from build123d import *

# Parameters (mm, degrees)
SALIENTE_EXTRUIR1_DEPTH  = 67.25
CROQUIS7_R               = 4
SALIENTE_EXTRUIR2_DEPTH  = 15
SALIENTE_EXTRUIR9_DEPTH  = 7.5
CROQUIS15_R              = 4
SALIENTE_EXTRUIR15_DEPTH = 9
CROQUIS17_W              = 25
CROQUIS17_H              = 5
SALIENTE_EXTRUIR16_DEPTH = 17.5
CROQUIS18_R              = 1.75
CORTAR_EXTRUIR3_DEPTH    = 7.5


with BuildPart() as part:
    # Croquis2 → Saliente-Extruir1 (new body)
    with BuildSketch(Plane(origin=(0, 0, 0), x_dir=(1, 0, 0), z_dir=(0, 1, 0))):
        Polygon((-17.5, -27.121137051), (17.5, -27.121137051), (17.5, -17.121137051), (9.5, -17.121137051), (9.5, -14.121137051), (17.5, -14.121137051), (7.5, -4.121137051), (-7.5, -4.121137051), (-17.5, -14.121137051), (-9.5, -14.121137051), (-9.5, -17.121137051), (-17.5, -17.121137051), align=None)
    extrude(amount=SALIENTE_EXTRUIR1_DEPTH)

    # Croquis7 → Saliente-Extruir2 (add)
    with BuildSketch(Plane.XY.offset(27.121137051)):
        with Locations(Location((0, 54.15, 0), (0, 0, 180))):
            Circle(CROQUIS7_R)
    extrude(amount=SALIENTE_EXTRUIR2_DEPTH)



with BuildPart() as body_2:
    # Croquis8 → Saliente-Extruir9 (new, symmetric)
    with BuildSketch(Plane(origin=(0, 0, 0), x_dir=(0, 0, -1), z_dir=(1, 0, 0))):
        Polygon((-36.121137051, 47.65), (-30.523413607, 47.65), (-27.121137051, 47.65), (-27.121137051, 37.610022974), align=None)
    extrude(amount=SALIENTE_EXTRUIR9_DEPTH, both=True)


with BuildPart() as part_1:
    add(part.part)

    add(body_2.part)  # Saliente-Extruir15 merges body 2
    # Croquis15 → Saliente-Extruir15 (add)
    with BuildSketch(Plane.XY.offset(27.121137051)):
        with BuildLine():
            Line((-7.5, 47.65), (7.5, 47.65))
            Line((7.5, 47.65), (7.5, 57.15))
            ThreePointArc((7.5, 57.15), (6.474873734, 59.624873734), (4, 60.65))
            Line((4, 60.65), (-4, 60.65))
            ThreePointArc((-4, 60.65), (-6.474873734, 59.624873734), (-7.5, 57.15))
            Line((-7.5, 57.15), (-7.5, 47.65))
        make_face()
        with Locations(Location((0, 54.15, 0), (0, 0, 180))):
            Circle(CROQUIS15_R, mode=Mode.SUBTRACT)
    extrude(amount=SALIENTE_EXTRUIR15_DEPTH)

    # Croquis17 → Saliente-Extruir16 (add, symmetric)
    with BuildSketch(Plane(origin=(0, 0, 0), x_dir=(0, 0, -1), z_dir=(1, 0, 0))):
        with Locations((-39.621137051, 5.5)):
            Rectangle(CROQUIS17_W, CROQUIS17_H)
    extrude(amount=SALIENTE_EXTRUIR16_DEPTH, both=True)

    # Croquis18 → Cortar-Extruir3 (cut, symmetric)
    with BuildSketch(Plane(origin=(0, 8, 0), x_dir=(1, 0, 0), z_dir=(0, 1, 0))):
        with Locations(Location((0, -47.121137051, 0), (0, 0, 270))):
            Circle(CROQUIS18_R)
    extrude(amount=CORTAR_EXTRUIR3_DEPTH, both=True, mode=Mode.SUBTRACT)


solid = part_1.part
Model file for the job. Use its own axes, mm. A direction names the side the tool comes from. Give positions to 0.01 mm unless a question says otherwise; leave off trailing zeros. Loops run counter-clockwise (first coordinate to the right, second up) from the corner with the lowest first, then second, coordinate; pieces in that order, holes last. Notation, with made-up numbers: (67.25, -21) -> (123.25, -21) arc R20 ccw to (123.25, -1) -> close; hole circle Ø6 at (-6, 86.25). An arc over 180 degrees is marked (long way). Use a Markdown table: item, result. Add a question column.
(1) Slice it at D-D on z = 44. List the corners of the cut face in (x, y).
(2) Tool access for faces 5 (the flat face through (0, 54, 42.121)), 6 (the flat face through (9.5, 33, 16)), 7 (the cylindrical face through (-6.4, 59.7, 31.6)): list every direction of +Z, -Z, +X, -X, +Y, -Y with a clear straight run to the whole face (end or side of a thin tool).
(3) Slice it at B-B on y = 54.15. List the corners of the cut face in (x, z).
(4) Mould opens along Z. For faces 1 (the flat face through (-7.5, 50, 32)), 2 (the flat face through (0.11, 42.56, 31.56)), 3 (the cylindrical face through (-0.67, 5.535, 48.738)), 4 (the flat face through (0, 33, 4.121)) say: +Z half, -Z half, draft (parallel to the pull), parting line (faces both ways), or undercut.
(5) Slice it at C-C on y = 7. List the corners of the cut face in (x, z), and give its area (3 significant figures).
(6) Drop flat-ended pins along their axis: pin 1 Ø10 at (x, z) = (-8.5, 36.5) entering from +Y; pin 2 Ø0.9 at (y, z) = (50, 15) entering from +X; pin 3 Ø6 at (x, z) = (-5.5, 39) entering from -Y. Give the stop position or say it passes through.
(7) Wall check: line 1 along Y through (x, z) = (-14, 45.5); line 2 along X through (y, z) = (49, 17); line 3 along Z through (x, y) = (-13, 28.5). Give the ranges that are in metal, low to high.
(8) Slice it at A-A on x = -11. List the corners of the cut face in (y, z), and give its area (3 significant figures).
Filled sheet:
| question | item | result |
|---|---|---|
| 1 | outline | (-17.5, 3) -> (17.5, 3) -> (17.5, 8) -> (-17.5, 8) -> close |
| 2 | face 5 | +Z, +X, -X, +Y |
| 2 | face 6 | +X, +Y, -Y |
| 2 | face 7 | +Z, -X, +Y |
| 3 | outline | (-17.5, 14.12) -> (-7.5, 4.12) -> (7.5, 4.12) -> (17.5, 14.12) -> (9.5, 14.12) -> (9.5, 17.12) -> (17.5, 17.12) -> (17.5, 27.12) -> (7.5, 27.12) -> (7.5, 36.12) -> (4, 36.12) -> (4, 42.12) -> (-4, 42.12) -> (-4, 36.12) -> (-7.5, 36.12) -> (-7.5, 27.12) -> (-17.5, 27.12) -> (-17.5, 17.12) -> (-9.5, 17.12) -> (-9.5, 14.12) -> close |
| 4 | face 1 | draft |
| 4 | face 2 | +Z half |
| 4 | face 3 | undercut |
| 4 | face 4 | -Z half |
| 5 | outline | (-17.5, 14.12) -> (-7.5, 4.12) -> (7.5, 4.12) -> (17.5, 14.12) -> (9.5, 14.12) -> (9.5, 17.12) -> (17.5, 17.12) -> (17.5, 52.12) -> (-17.5, 52.12) -> (-17.5, 17.12) -> (-9.5, 17.12) -> (-9.5, 14.12) -> close; hole circle Ø3.5 at (0, 47.12) |
| 5 | area | 1,520 mm2 |
| 6 | pin 1 | y = 60.65 |
| 6 | pin 2 | x = 9.5 |
| 6 | pin 3 | y = 3 |
| 7 | line 1 | 3 to 8 |
| 7 | line 2 | -9.5 to 9.5 |
| 7 | line 3 | 9.62 to 14.12, 17.12 to 27.12 |
| 8 | outline | (0, 7.62) -> (67.25, 7.62) -> (67.25, 14.12) -> (0, 14.12) -> close; (0, 17.12) -> (67.25, 17.12) -> (67.25, 27.12) -> (8, 27.12) -> (8, 52.12) -> (3, 52.12) -> (3, 27.12) -> (0, 27.12) -> close |
| 8 | area | 1,230 mm2 |
